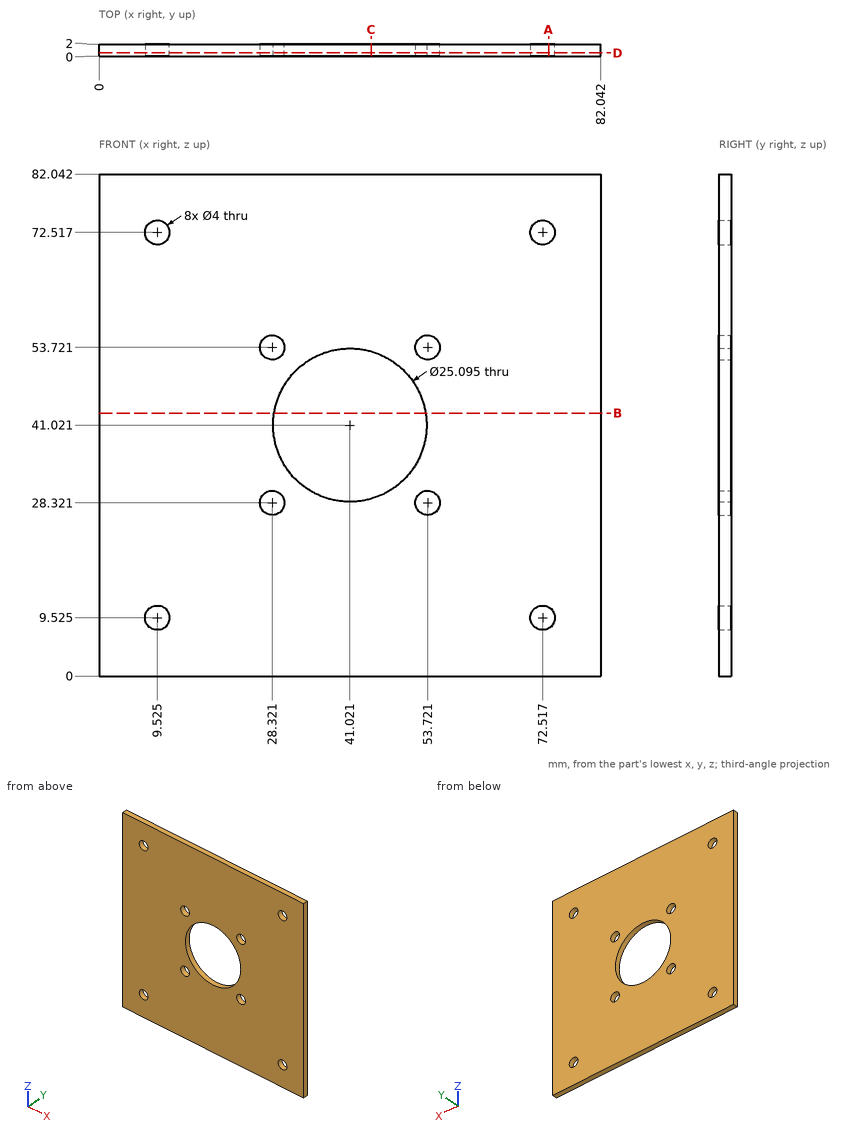
Drawing for the job (mm, zero at the part's lowest x, y, z). Round coordinates to 2 decimals unless told otherwise and drop trailing zeros. Write each loop counter-clockwise with the first axis right and the second up, starting at its lowest first coordinate (ties: lowest second). Pieces come first, ordered by that corner, then holes.
Item 1: Band-saw the part on D-D on y = 0.55. Give the number of separate pieces and of enclosed holes in the cut face, then the cut area to 3 significant figures.
Filled in:
separate pieces: 1
enclosed holes: 9
area: 6,140 mm2
Item 2: Band-saw the part on B-B on z = 43. Write the cut outline in (x, y).
Filled in:
outline: (0, 0) - (28.63, 0) - (28.63, 2) - (0, 2) - close; (53.41, 0) - (82.04, 0) - (82.04, 2) - (53.41, 2) - close
Item 3: Drill centre lines: L1, parallel to X at y = 1.85, z = 55.5 (1 decimal); L2, parallel to X at y = 0.3, z = 41.5; L3, parallel to X at y = 0.4, z = 73.5 (1 decimal). Where is each one in solid material? Low to high.
Filled in:
L1: x = 0 to 27.4, 29.2 to 52.8, 54.6 to 82
L2: x = 0 to 28.48, 53.56 to 82.04
L3: x = 0 to 7.8, 11.3 to 70.8, 74.3 to 82
Item 4: Band-saw the part on A-A on x = 73.5. Write the cut outline in (y, z) (1 decimal), then the cut area to 3 significant figures.
Filled in:
outline: (0, 0) - (2, 0) - (2, 7.8) - (0, 7.8) - close; (0, 11.3) - (2, 11.3) - (2, 70.8) - (0, 70.8) - close; (0, 74.3) - (2, 74.3) - (2, 82) - (0, 82) - close
area: 150 mm2
Item 5: Band-saw the part on C-C on x = 44.5. Write the cut outline in (y, z) (1 decimal), then the cut area to 3 significant figures.
Filled in:
outline: (0, 0) - (2, 0) - (2, 29) - (0, 29) - close; (0, 53.1) - (2, 53.1) - (2, 82) - (0, 82) - close
area: 116 mm2
